```python
from build123d import *

# Parameters (mm, degrees)
CIRCLE070_R        = 12
EXTRUSION013_DEPTH = 4
CIRCLE066_R        = 11
EXTRUSION012_DEPTH = 14
CIRCLE_R           = 13
EXTRUSION_DEPTH    = 14.5
CIRCLE069_R        = 9
EXTRUDE072_DEPTH   = 2
CIRCLE067_R        = 3
EXTRUDE_DEPTH      = 11
CIRCLE068_R        = 5
EXTRUDE071_DEPTH   = 11


with BuildPart() as extrusion013:
    # Circle070 → Extrusion013 (new body)
    with BuildSketch(Plane(origin=(-85.118271, -1.008042, 9), x_dir=(1, 0, 0), z_dir=(0, 0, 1))):
        Circle(CIRCLE070_R)
    extrude(amount=EXTRUSION013_DEPTH)


with BuildPart() as extrusion013_1:
    # Extrusion013 placement: moved
    add(extrusion013.part.moved(Location((26.958331, 4.39901, 0.5))))


with BuildPart() as extrusion012:
    # Circle066 → Extrusion012 (new body)
    with BuildSketch(Plane(origin=(17.627983, 9.639136, 13.765504), x_dir=(1, 0, 0), z_dir=(0, 0, 1))):
        Circle(CIRCLE066_R)
    extrude(amount=-EXTRUSION012_DEPTH)


with BuildPart() as cut048:
    # Circle → Extrusion (new body)
    with BuildSketch(Plane(origin=(17.627983, 9.639136, -0.734496), x_dir=(1, 0, 0), z_dir=(0, 0, -1))):
        Circle(CIRCLE_R)
    extrude(amount=-EXTRUSION_DEPTH)

    # Cut: cut Extrusion012
    add(extrusion012.part, mode=Mode.SUBTRACT)


with BuildPart() as cut048_1:
    # Cut placement: moved
    add(cut048.part.moved(Location((-75.787923, -6.248169, 9.734496))))

    # Cut048: cut Extrusion013
    add(extrusion013_1.part, mode=Mode.SUBTRACT)


with BuildPart() as extrude072:
    # Circle069 → Extrude072 (new body)
    with BuildSketch(Plane(origin=(-58.15994, 3.390968, 9), x_dir=(1, 0, 0), z_dir=(0, 0, -1))):
        Circle(CIRCLE069_R)
    extrude(amount=-EXTRUDE072_DEPTH)


with BuildPart() as extrude_body:
    # Circle067 → Extrude (new body)
    with BuildSketch(Plane(origin=(-58.15994, 3.390968, 9), x_dir=(1, 0, 0), z_dir=(0, 0, -1))):
        Circle(CIRCLE067_R)
    extrude(amount=-EXTRUDE_DEPTH)


with BuildPart() as fusion001:
    # Circle068 → Extrude071 (new body)
    with BuildSketch(Plane(origin=(-58.15994, 3.390968, 9), x_dir=(1, 0, 0), z_dir=(0, 0, -1))):
        Circle(CIRCLE068_R)
    extrude(amount=-EXTRUDE071_DEPTH)

    # Cut047: cut Extrude body
    add(extrude_body.part, mode=Mode.SUBTRACT)

    # Fusion: union Extrude072
    add(extrude072.part)

    # Fusion001: union Cut048
    add(cut048_1.part)


solid = fusion001.part
```
Read the model definition and answer for the solid it produces. Units are mm, in the model's axes. A direction names the side the tool comes from. Coordinates: 2 decimals unless noted, no trailing zeros. Write each loop counter-clockwise with the first axis right and the second up, starting at its lowest first coordinate (ties: lowest second). Pieces come first, ordered by that corner, then holes. Notation, with made-up numbers: (32.25, 65) -> (48.25, 65) arc R18 ccw to (48.25, 78) -> close; hole circle Ø7 at (39, 16). An arc over 180 degrees is marked (long way). Write item = value, one per line.
(1) Which of the six approach directions +Z, -Z, +X, -X, +Y, -Y give full straight-line access (tool end or side, diameter ignored) to faces 1 (the face through (-58, 3, 9)), 2 (the face through (-48, -2, 13.5)), 3 (the face through (-54, 7, 11))?
From the geometry:
face_1 = -Z, +X, -X, +Y, -Y
face_2 = none
face_3 = +Z
(2) Given pin 1 Ø1.5 at (y, z) = (-2.5, 15) entering from +X; pin 2 Ø13 at (x, y) = (-58.16, 3.39) entering from +Z; pin 3 Ø1 at (y, z) = (0, 19.5) entering from -X, each flat-ended and moving along its own axis, determine where each tip first touches the part or whether it passes through.
From the geometry:
pin_1 = -46.22
pin_2 = 20
pin_3 = -70.83
(3) Section B-B on x = -54.75 is taken. Write down the section's boundary in (y, z).
From the geometry:
outline = (-9.15, 9) -> (15.94, 9) -> (15.94, 23.5) -> (13.85, 23.5) -> (13.85, 13.5) -> (14.9, 13.5) -> (14.9, 9.5) -> (11.72, 9.5) -> (11.72, 11) -> (7.05, 11) -> (7.05, 20) -> (-0.27, 20) -> (-0.27, 11) -> (-4.94, 11) -> (-4.94, 9.5) -> (-8.11, 9.5) -> (-8.11, 13.5) -> (-7.07, 13.5) -> (-7.07, 23.5) -> (-9.15, 23.5) -> close
(4) Section C-C on y = -1 is taken. Write down the section's boundary in (x, z), plus the area to 3 significant figures.
From the geometry:
outline = (-70.4, 9) -> (-45.92, 9) -> (-45.92, 23.5) -> (-48.07, 23.5) -> (-48.07, 13.5) -> (-46.99, 13.5) -> (-46.99, 9.5) -> (-50.3, 9.5) -> (-50.3, 11) -> (-55.77, 11) -> (-55.77, 20) -> (-60.55, 20) -> (-60.55, 11) -> (-66.02, 11) -> (-66.02, 9.5) -> (-69.33, 9.5) -> (-69.33, 13.5) -> (-68.25, 13.5) -> (-68.25, 23.5) -> (-70.4, 23.5) -> close
area = 130 mm2
(5) For a pull along Y with two mould halves and no side action, classify faces 4 (the face through (-45.76, -0.51, 16.15)), 5 (the face through (-53.39, 1.89, 15.44)), 6 (the face through (-69, 0, 23.5)) as +Y half, -Y half, draft (parallel to the pull), parting line (faces both ways), or undercut.
From the geometry:
face_4 = parting line
face_5 = undercut
face_6 = draft
(6) Straight lines are drawn through the part: L1, parallel to Y at x = -58, z = 11.25; L2, parallel to X at y = 1.5, z = 16.75; L3, parallel to Y at x = -56, z = 13.75. For each, find the intervals that lie inside material, in ascending order. Write a range as from..to.
From the geometry:
L1 = -9.61..-8.61, -1.61..0.4, 6.39..8.39, 15.39..16.39
L2 = -71.02..-69, -62.79..-60.49, -55.83..-53.53, -47.32..-45.3
L3 = -9.43..-7.39, -1.12..1.31, 5.47..7.9, 14.18..16.21
(7) Section A-A on z = 14.25 is taken. Write down the section's boundary in (x, y), plus the area to 3 significant figures.
From the geometry:
outline = circle Ø26 at (-58.16, 3.39); circle Ø10 at (-58.16, 3.39); hole circle Ø22 at (-58.16, 3.39); hole circle Ø6 at (-58.16, 3.39)
area = 201 mm2
(8) Section D-D on x = -64.5 is taken. Write down the section's boundary in (y, z), plus the area to 3 significant figures.
From the geometry:
outline = (-7.96, 9) -> (14.74, 9) -> (14.74, 23.5) -> (12.38, 23.5) -> (12.38, 13.5) -> (13.58, 13.5) -> (13.58, 9.5) -> (9.78, 9.5) -> (9.78, 11) -> (-3, 11) -> (-3, 9.5) -> (-6.8, 9.5) -> (-6.8, 13.5) -> (-5.6, 13.5) -> (-5.6, 23.5) -> (-7.96, 23.5) -> close
area = 87.0 mm2
